from build123d import *

# Parameters (mm, degrees)
CYLINDER001_R     = 9.5
CYLINDER001_DEPTH = 153
CYLINDER_R        = 11
CYLINDER_DEPTH    = 153
CUT_PITCH_ANGLE   = 90


with BuildPart() as int:
    # Cylinder001 → Cylinder001 (new body)
    with BuildSketch(Plane.XY.offset(2.5)):
        Circle(CYLINDER001_R)
    extrude(amount=CYLINDER001_DEPTH)


with BuildPart() as steeltube:
    # Cylinder → Cylinder (new body)
    with BuildSketch(Plane.XY.offset(2.5)):
        Circle(CYLINDER_R)
    extrude(amount=CYLINDER_DEPTH)

    # Cut: cut INT
    add(int.part, mode=Mode.SUBTRACT)


with BuildPart() as steeltube_1:
    # Cut pitch: moved
    add(steeltube.part.rotate(Axis((0, 0, 0), (0, 1, 0)), CUT_PITCH_ANGLE))


with BuildPart() as steeltube_2:
    # Cut placement: moved
    add(steeltube_1.part)


solid = steeltube_2.part
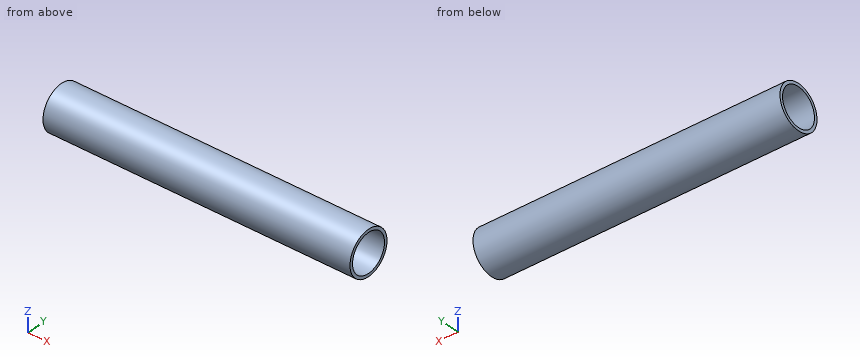
The listing builds one solid part. Answer for the finished solid, in the listing's coordinates (mm). Round coordinates to 2 decimals unless told otherwise and drop trailing zeros. Write each loop counter-clockwise with the first axis right and the second up, starting at its lowest first coordinate (ties: lowest second). Pieces come first, ordered by that corner, then holes. Notation, with made-up numbers: (25.25, 61.25) - (66.25, 61.25) arc R22 cw to (66.25, 92.25) - close; hole circle Ø7 at (32.25, 79). An arc over 180 degrees is marked (long way). Use a Markdown table: item, result. Add a question column.
1. Consider line 1 (Z direction, x = 149, y = 0.5); line 2 (Y direction, x = 80, z = 0); line 3 (Z direction, x = 121, y = -8). Determine where each line is inside the solid, lowest interval first.
2. Flat-ended cylindrical pins translate along their axes: P1, Ø3, axis at x = 57.5, y = 6, coming from the -Z side; P2, Ø3, axis at x = 24.5, z = 8.5, coming from the +Y side; P3, Ø6, axis at x = 91, y = -8.5, coming from the -Z side. Find the tip coordinate at first contact, or state that the pin passes through.
3. The part is cut by section C-C (x = 83.5). Write down the section's boundary in (y, z).
4. The part is cut by section A-A (z = 0). Write down the section's boundary in (x, y).
Reported:
| question | item | result |
|---|---|---|
| 1 | line 1 | -10.99 to -9.49, 9.49 to 10.99 |
| 1 | line 2 | -11 to -9.5, 9.5 to 11 |
| 1 | line 3 | -7.55 to -5.12, 5.12 to 7.55 |
| 2 | P1 | z = -10.04 |
| 2 | P2 | y = 8.49 |
| 2 | P3 | z = -9.53 |
| 3 | outline | circle Ø22 at (0, 0); hole circle Ø19 at (0, 0) |
| 4 | outline | (2.5, -11) - (155.5, -11) - (155.5, -9.5) - (2.5, -9.5) - close; (2.5, 9.5) - (155.5, 9.5) - (155.5, 11) - (2.5, 11) - close |
